For this review, use the dimensioned drawing (mm, ordinates from the lowest corner) and the shaded views. A direction names the side the tool comes from. Round coordinates to 2 decimals unless told otherwise and drop trailing zeros. Write each loop counter-clockwise with the first axis right and the second up, starting at its lowest first coordinate (ties: lowest second). Pieces come first, ordered by that corner, then holes. Notation, with made-up numbers: (19, 79) -> (70, 79) arc R23 cw to (70, 115) -> close; hole circle Ø8 at (81, 78). An arc over 180 degrees is marked (long way). Answer in a Markdown table with one row per item. Add a question column.
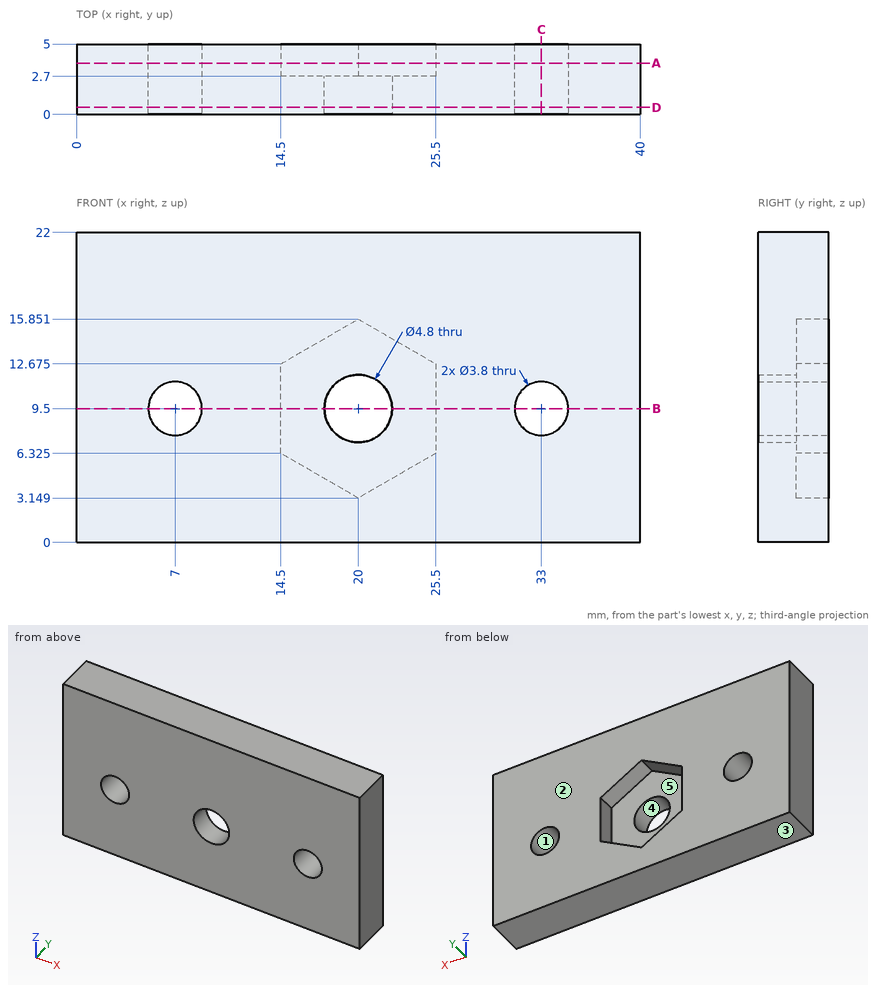
1. We need section B-B (z = 9.5). Write out the cut boundary in (x, y).
2. We need section C-C (x = 33). Write out the cut boundary in (y, z), plus the area to 3 significant figures.
3. We need section D-D (y = 0.5). Write out the cut boundary in (x, z), plus the area to 3 significant figures.
4. For L1, parallel to Z at x = 33, y = 3.3; L2, parallel to X at y = 4, z = 6.75; L3, parallel to Y at x = 17, z = 12.5, list the stretches that pass through material, from the lowest coordinate up. Write a range as [from, to].
5. Tool access review of the marked faces 4 and 5: name each direction out of +Z, -Z, +X, -X, +Y, -Y from which nothing blocks a thin tool from reaching the whole face with its end or side.
6. We need section A-A (y = 3.65). Count the separate pieces of the cut face and the enclosed holes in it.
7. The part is to be moulded in two halves that separate along Z. For the marked faces 1, 2 and 3, say which applies: pulls with the +Z half, pulls with the -Z half, needs draft (parallel to the pull), parting line crosses it, or undercut.
8. Clearance check with a flat-ended pin moving along its axis: pin 1 Ø3.5 at (x, z) = (20.5, 11) entering from +Y. State where the tip first meets the part, or that it passes through.
Response:
| question | item | result |
|---|---|---|
| 1 | outline | (0, 0) -> (5.1, 0) -> (5.1, 5) -> (0, 5) -> close; (8.9, 0) -> (17.6, 0) -> (17.6, 2.7) -> (14.5, 2.7) -> (14.5, 5) -> (8.9, 5) -> close; (22.4, 0) -> (31.1, 0) -> (31.1, 5) -> (25.5, 5) -> (25.5, 2.7) -> (22.4, 2.7) -> close; (34.9, 0) -> (40, 0) -> (40, 5) -> (34.9, 5) -> close |
| 2 | outline | (0, 0) -> (5, 0) -> (5, 7.6) -> (0, 7.6) -> close; (0, 11.4) -> (5, 11.4) -> (5, 22) -> (0, 22) -> close |
| 2 | area | 91.0 mm2 |
| 3 | outline | (0, 0) -> (40, 0) -> (40, 22) -> (0, 22) -> close; hole circle Ø3.8 at (7, 9.5); hole circle Ø4.8 at (20, 9.5); hole circle Ø3.8 at (33, 9.5) |
| 3 | area | 839 mm2 |
| 4 | L1 | [0, 7.6], [11.4, 22] |
| 4 | L2 | [0, 14.5], [25.5, 40] |
| 4 | L3 | [0, 2.7] |
| 5 | face 4 | +Y, -Y |
| 5 | face 5 | +Y |
| 6 | separate pieces | 1 |
| 6 | enclosed holes | 3 |
| 7 | face 1 | undercut |
| 7 | face 2 | needs draft |
| 7 | face 3 | pulls with the -Z half |
| 8 | pin 1 | y = 2.7 |
